Answer from the drawing. Dimensions are ordinates in mm from the lowest x, y and z of the part. A direction names the side the tool comes from. Round coordinates to 2 decimals unless told otherwise and drop trailing zeros. Order: outer loops, then holes, each group sorted by start corner. A loop starts at its lowest first (then second) coordinate and runs counter-clockwise, first axis right, second up. Notation, with made-up numbers: (48, 69) -> (56, 69) arc R22 ccw to (56, 105) -> close; hole circle Ø1 at (87.25, -3.75). An arc over 180 degrees is marked (long way). Use a Markdown table: item, result. Add a question column.
Item 1: A cutting plane is placed at C-C, the plane x = 65. Determine the outline of the cut face in (y, z), plus the area to 3 significant figures.
Item 2: A cutting plane is placed at B-B, the plane y = 60. Determine the outline of the cut face in (x, z).
Item 3: Flat-ended cylindrical pins translate along their axes: P1, Ø18.5, axis at x = 65, y = 35, coming from the +Z side; P2, Ø5.5, axis at x = 85, z = 2.5, coming from the -Y side; P3, Ø5, axis at x = 108.5, z = 3.5, coming from the +Y side. Find the tip coordinate at first contact, or state that the pin passes through.
Item 4: For a pull along X with two mould halves and no side action, classify the marked faces 1, 2 and 3 as +X half, -X half, draft (parallel to the pull), parting line (faces both ways), or undercut.
Item 5: A cutting plane is placed at A-A, the plane z = 13.5. Determine the outline of the cut face in (x, y), plus the area to 3 significant figures.
Item 6: Find the intervals of material crossed by L1, parallel to Y at x = 128.9, z = 20; L2, parallel to Y at x = 65, z = 0.8; L3, parallel to Z at x = 128, y = 10, in increasing order. Write a range as [from, to].
Item 7: A cutting plane is placed at D-D, the plane z = 20. Determine the outline of the cut face in (x, y), plus the area to 3 significant figures.
Item 8: A tool of negligible diameter and unlimited length cuts with its end or side. For the marked faces 4 and 5, from which of +Z, -Z, +X, -X, +Y, -Y can it reach the whole face along a straight path? Write none if from no direction.
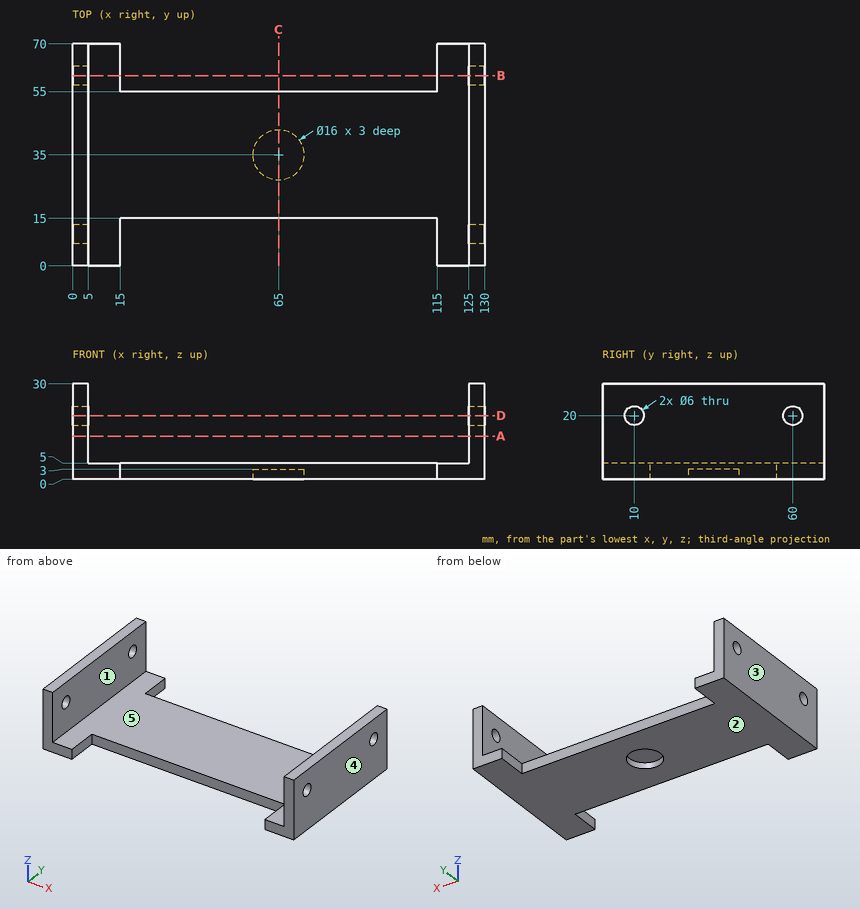
Reported:
| question | item | result |
|---|---|---|
| 1 | outline | (15, 0) -> (27, 0) -> (27, 3) -> (43, 3) -> (43, 0) -> (55, 0) -> (55, 5) -> (15, 5) -> close |
| 1 | area | 152 mm² |
| 2 | outline | (0, 0) -> (15, 0) -> (15, 5) -> (5, 5) -> (5, 17) -> (0, 17) -> close; (0, 23) -> (5, 23) -> (5, 30) -> (0, 30) -> close; (115, 0) -> (130, 0) -> (130, 17) -> (125, 17) -> (125, 5) -> (115, 5) -> close; (125, 23) -> (130, 23) -> (130, 30) -> (125, 30) -> close |
| 3 | P1 | z = 5 |
| 3 | P2 | y = 15 |
| 3 | P3 | y = 55 |
| 4 | face 1 | undercut |
| 4 | face 2 | draft |
| 4 | face 3 | -X half |
| 5 | outline | (0, 0) -> (5, 0) -> (5, 70) -> (0, 70) -> close; (125, 0) -> (130, 0) -> (130, 70) -> (125, 70) -> close |
| 5 | area | 700 mm² |
| 6 | L1 | [0, 7], [13, 57], [63, 70] |
| 6 | L2 | [15, 27], [43, 55] |
| 6 | L3 | [0, 17], [23, 30] |
| 7 | outline | (0, 0) -> (5, 0) -> (5, 7) -> (0, 7) -> close; (0, 13) -> (5, 13) -> (5, 57) -> (0, 57) -> close; (0, 63) -> (5, 63) -> (5, 70) -> (0, 70) -> close; (125, 0) -> (130, 0) -> (130, 7) -> (125, 7) -> close; (125, 13) -> (130, 13) -> (130, 57) -> (125, 57) -> close; (125, 63) -> (130, 63) -> (130, 70) -> (125, 70) -> close |
| 7 | area | 580 mm² |
| 8 | face 4 | +Z, -Z, +X, +Y, -Y |
| 8 | face 5 | +Z, +Y, -Y |
